Design review of the part built by this model. Coordinates are the model's own, in mm. A direction names the side the tool comes from. Coordinates: 2 decimals unless noted, no trailing zeros. Loops run counter-clockwise (first coordinate to the right, second up) from the corner with the lowest first, then second, coordinate; pieces in that order, holes last. Notation, with made-up numbers: M -35.75,-11 L 8.25,-11 A28 cw 8.25,28 Z; hole C 3,-17.75 d5. An arc over 180 degrees is marked long. Put each result on its own line as item: value. Start each with the question number.
(1) The part is to be moulded in two halves that separate along X. For faces 1 (the cylindrical face through (-19.176, 0.066, 8.521)), 2 (the cylindrical face through (-8.4, -37.83, 4.93)), 3 (the flat face through (19.9, -31.4, 0)), 4 (the cylindrical face through (0.806, -16.413, 8.521)), say which applies: +X half, -X half, draft (parallel to the pull), parting line (faces both ways), or undercut.
(2) For probe 1 along Y at (x, z) = (0, 9.15); probe 2 along Z at (x, y) = (-12, -22.5); probe 3 along X at (y, z) = (-8.5, 0.5), list the stretches that pass through material, from the lowest coordinate up. Write a range as [from, to].
(3) Clearance check with flat-ended pins moving along their axes: pin 1 (3 mm diameter, centred on x = 10, z = 5, fed in from +Y); pin 2 (3.5 mm diameter, centred on x = 0, y = -17.68, fed in from -Z); pin 3 (6 mm diameter, centred on y = -14, z = 2, fed in from -X). State where each tip first meets the part, or that it passes through.
(4) Take a section at C-C, the plane z = 2.5. Give the boundary of the cut face in (x, y), then the cut area to 3 significant figures.
(5) Take a section at A-A, the plane x = 0. Give the boundary of the cut face in (y, z), then the cut area to 3 significant figures.
(6) Take a section at D-D, the plane y = -29. Give the boundary of the cut face in (x, z), then the cut area to 3 significant figures.
(7) For faces 5 (the cylindrical face through (2.17, -9.76, 6.51)), 6 (the cylindrical face through (16.18, 0.07, 8.52)), list the 3-axis set-ups (+Z, -Z, +X, -X, +Y, -Y) from which the entire face can be reached by the end or side of a thin tool; tool diameter is ignored.
```python
from build123d import *

# Parameters (mm, degrees)
SKETCH_1_R          = 38.75
EXTRUDE_1_DEPTH     = 10
SKETCH_2_R          = 37
CUT_EXTRUDE_1_DEPTH = 7
SKETCH_3_R          = 10
EXTRUDE_2_DEPTH     = 1
SKETCH_4_R          = 1.5
CUT_EXTRUDE_2_DEPTH = 56.705699888


with BuildPart() as part:
    # 草图1 → 凸台-拉伸1 (new body)
    with BuildSketch(Plane.XY):
        Circle(SKETCH_1_R)
    extrude(amount=EXTRUDE_1_DEPTH)

    # 草图2 → 切除-拉伸1 (cut)
    with BuildSketch(Plane(origin=(0, 0, 0), x_dir=(-1, 0, 0), z_dir=(0, 0, -1))):
        Circle(SKETCH_2_R)
    extrude(amount=-CUT_EXTRUDE_1_DEPTH, mode=Mode.SUBTRACT)

    # 草图3 → 凸台-拉伸2 (add)
    with BuildSketch(Plane(origin=(0, 0, 7), x_dir=(-1, 0, 0), z_dir=(0, 0, -1))):
        Circle(SKETCH_3_R)
    extrude(amount=EXTRUDE_2_DEPTH)

    # 草图4 → 切除-拉伸2 (cut, through all)
    with BuildSketch(Plane.XY.offset(10)):
        with Locations((0, 17.67766953)):
            Circle(SKETCH_4_R)
        with Locations((17.67766953, 0)):
            Circle(SKETCH_4_R)
        with Locations((0, -17.67766953)):
            Circle(SKETCH_4_R)
        with Locations((-17.67766953, 0)):
            Circle(SKETCH_4_R)
        Circle(SKETCH_4_R)
    extrude(amount=-CUT_EXTRUDE_2_DEPTH, mode=Mode.SUBTRACT)


solid = part.part
```
Computed values:
1. face 1: undercut
1. face 2: parting line
1. face 3: draft
1. face 4: undercut
2. probe 1: y = [-38.75, -19.18], [-16.18, -1.5], [1.5, 16.18], [19.18, 38.75]
2. probe 2: z = [7, 10]
2. probe 3: x = [-37.81, -36.01], [36.01, 37.81]
3. pin 1: stops at y = 37.81
3. pin 2: stops at z = 7
3. pin 3: stops at x = -37.16
4. outline: C 0,0 d77.5; hole C 0,0 d74
4. area: 416 mm^2
5. outline: M -38.75,0 L -37,0 L -37,7 L -19.18,7 L -19.18,10 L -38.75,10 Z; M -16.18,7 L -10,7 L -10,6 L -1.5,6 L -1.5,10 L -16.18,10 Z; M 1.5,6 L 10,6 L 10,7 L 16.18,7 L 16.18,10 L 1.5,10 Z; M 19.18,7 L 37,7 L 37,0 L 38.75,0 L 38.75,10 L 19.18,10 Z
5. area: 247 mm^2
6. outline: M -25.7,0 L -22.98,0 L -22.98,7 L 22.98,7 L 22.98,0 L 25.7,0 L 25.7,10 L -25.7,10 Z
6. area: 192 mm^2
7. face 5: -Z
7. face 6: +Z, -Z
